```python
from build123d import *

# Parameters (mm, degrees)
F2_DEPTH = 4.7


with BuildPart() as f2:
    # F1 (on Front) → F2 (new body)
    with BuildSketch(Plane.XZ):
        with BuildLine():
            Line((-15.3, 0), (0, 0))
            Line((0, 0), (0, 107.2981178668))
            ThreePointArc((0, 107.2981178668), (-1.4644660941, 110.8336517727), (-5, 112.2981178668))
            Line((-5, 112.2981178668), (-8.6609683494, 112.2981178668))
            ThreePointArc((-8.6609683494, 112.2981178668), (-9.9544197878, 112.1279194545), (-11.1598138738, 111.6289112173))
            Line((-11.1598138738, 111.6289112173), (-27.3231734022, 102.3027357692))
            Line((-27.3231734022, 102.3027357692), (-17.3277913046, 84.979562367))
            Line((-17.3277913046, 84.979562367), (-21.3987370541, 82.630647574))
            Line((-21.3987370541, 82.630647574), (-31.3941191517, 99.9538209762))
            Line((-31.3941191517, 99.9538209762), (-188.4631123523, 9.3258184573))
            ThreePointArc((-188.4631123523, 9.3258184573), (-190.794240786, 3.7022174784), (-185.9655997989, -0.0049747155))
            Line((-185.9655997989, -0.0049747155), (-159.4, -0.0120569506))
            Line((-159.4, -0.0120569506), (-159.4, -4.7120569506))
            Line((-159.4, -4.7120569506), (-154.7, -4.7120569506))
            Line((-154.7, -4.7120569506), (-154.7, -0.0120569506))
            Line((-154.7, -0.0120569506), (-154.7, 9.9879430494))
            Line((-154.7, 9.9879430494), (-150, 9.9879430494))
            Line((-150, 9.9879430494), (-150, -0.0120569506))
            Line((-150, -0.0120569506), (-150, -4.7120569506))
            Line((-150, -4.7120569506), (-145.3, -4.7120569506))
            Line((-145.3, -4.7120569506), (-145.3, -0.0120569506))
            Line((-145.3, -0.0120569506), (-29.4, -0.0120569506))
            Line((-29.4, -0.0120569506), (-29.4, -4.7120569506))
            Line((-29.4, -4.7120569506), (-24.7, -4.7120569506))
            Line((-24.7, -4.7120569506), (-24.7, -0.0113617169))
            Line((-24.7, -0.0113617169), (-24.7, 9.9886382831))
            Line((-24.7, 9.9886382831), (-20, 9.9886382831))
            Line((-20, 9.9886382831), (-20, 0))
            Line((-20, 0), (-20, -4.7006952337))
            Line((-20, -4.7006952337), (-15.3, -4.7006952337))
            Line((-15.3, -4.7006952337), (-15.3, 0))
        make_face()
    extrude(amount=F2_DEPTH)


solid = f2.part
```
Model file for the job. Use its own axes, mm. A direction names the side the tool comes from. Coordinates: 2 decimals unless noted, no trailing zeros. Loops run counter-clockwise (first coordinate to the right, second up) from the corner with the lowest first, then second, coordinate; pieces in that order, holes last. Notation, with made-up numbers: (50, 33.25) -> (74, 33.25) arc R13 cw to (74, 48.25) -> close; hole circle Ø11 at (13.5, 41.25). An arc over 180 degrees is marked (long way). Answer as a JSON object with one key per item and string values.
Q1. Flat gauge pins, fed straight in: P1, Ø2.5, axis at y = -3, z = -1.5, coming from the +X side; P2, Ø1, axis at x = -83, y = -1.5, coming from the +Z side; P3, Ø1.4, axis at x = -152.5, y = -1.5, coming from the -Z side. Where does each tip first touch, or does it go through?
Report:
{"P1": "stops at x = -15.3", "P2": "stops at z = 70.47", "P3": "stops at z = 9.99"}
Q2. Cut at D-D (x = -85.5). List the corners of the cut face in (y, z) (3 decimals).
Report:
{"outline": "(-4.7, -0.012) -> (0, -0.012) -> (0, 68.735) -> (-4.7, 68.735) -> close"}
Q3. 3-axis set-ups, long thin cutter, end or side, ignore diameter. For faces 4 (the flat face through (-8, -2, 0)), 5 (the flat face through (-18, -2, -4.701)), 6 (the flat face through (-145.3, -2, -2)): which of +Z, -Z, +X, -X, +Y, -Y reach the whole face in a straight line?
Report:
{"face 4": "-Z, +X, +Y, -Y", "face 5": "-Z, +X, -X, +Y, -Y", "face 6": "-Z, +Y, -Y"}
Q4. Probe probe 1 along Z at (x, y) = (-119, -0.2); probe 2 along Z at (x, y) = (-29, -4.15); probe 3 along X at (y, z) = (-1.85, 37). List the from-to ranges inside material, lowest first.
Report:
{"probe 1": "z = -0.01 to 49.41", "probe 2": "z = -4.71 to 95.8", "probe 3": "x = -140.5 to 0"}
Q5. Cut at C-C (y = -2.1). List the corners of the cut face in (x, z).
Report:
{"outline": "(-188.46, 9.33) arc R5 ccw to (-185.97, 0) -> (-159.4, -0.01) -> (-159.4, -4.71) -> (-154.7, -4.71) -> (-154.7, 9.99) -> (-150, 9.99) -> (-150, -4.71) -> (-145.3, -4.71) -> (-145.3, -0.01) -> (-29.4, -0.01) -> (-29.4, -4.71) -> (-24.7, -4.71) -> (-24.7, 9.99) -> (-20, 9.99) -> (-20, -4.7) -> (-15.3, -4.7) -> (-15.3, 0) -> (0, 0) -> (0, 107.3) arc R5 ccw to (-5, 112.3) -> (-8.66, 112.3) arc R5 ccw to (-11.16, 111.63) -> (-27.32, 102.3) -> (-17.33, 84.98) -> (-21.4, 82.63) -> (-31.39, 99.95) -> close"}
Q6. Cut at B-B (z = 3). List the corners of the cut face in (x, y).
Report:
{"outline": "(-190.55, -4.7) -> (-154.7, -4.7) -> (-154.7, 0) -> (-190.55, 0) -> close; (-150, -4.7) -> (-24.7, -4.7) -> (-24.7, 0) -> (-150, 0) -> close; (-20, -4.7) -> (0, -4.7) -> (0, 0) -> (-20, 0) -> close"}
Q7. Pull direction Z, two halves, no side cores. Call faces 1 (the flat face through (-7, -2, 112.298)), 2 (the flat face through (-26.326, -2.317, 91.171)), 3 (the flat face through (-76, -4.7, 42)): released by +Z, released by -Z, zero draft, split by the parting line, or undercut.
Report:
{"face 1": "released by +Z", "face 2": "undercut", "face 3": "zero draft"}
Q8. Cut at A-A (z = 96). List the corners of the cut face in (x, y).
Report:
{"outline": "(-38.25, -4.7) -> (-29.11, -4.7) -> (-29.11, 0) -> (-38.25, 0) -> close; (-23.69, -4.7) -> (0, -4.7) -> (0, 0) -> (-23.69, 0) -> close"}
